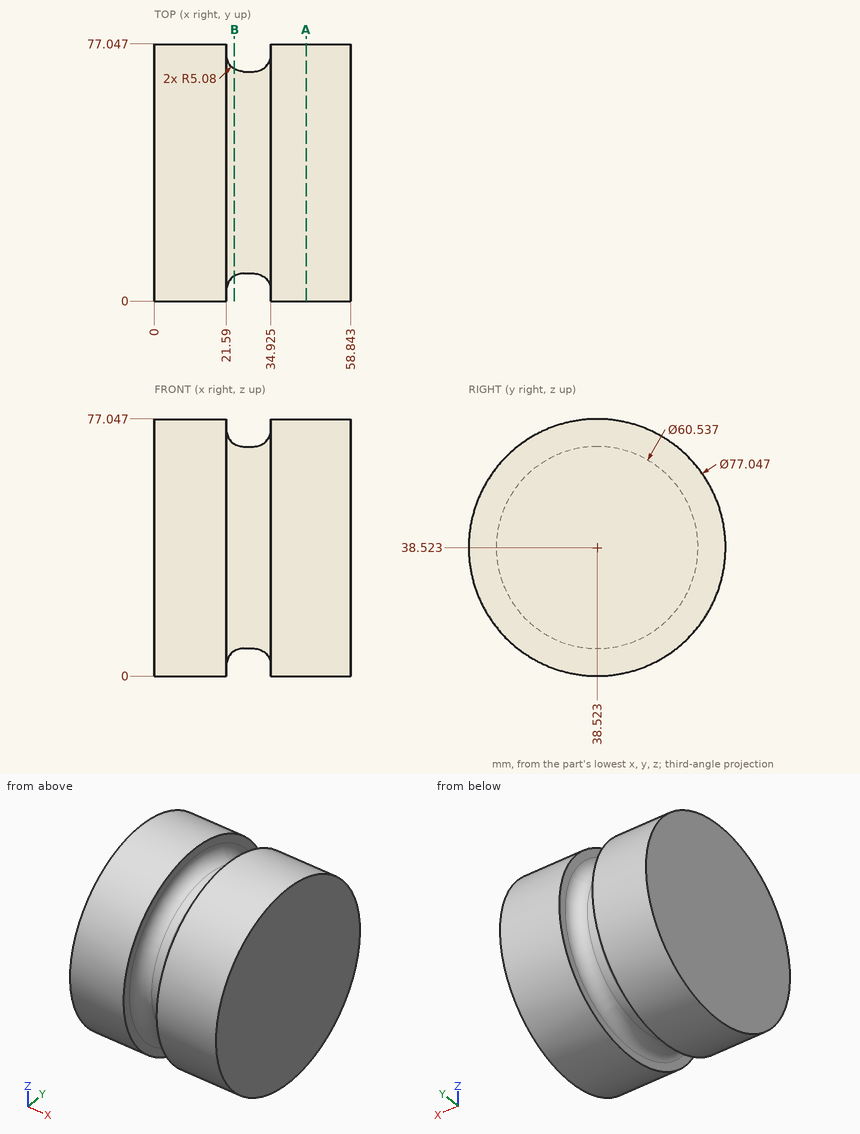
Print and shaded views of the part. All mm, measured from the part's lowest x, y and z. Give positions to 0.01 mm unless a question says otherwise; leave off trailing zeros. Write each loop counter-clockwise with the first axis right and the second up, starting at its lowest first coordinate (ties: lowest second). Pieces come first, ordered by that corner, then holes. Notation, with made-up numbers: M -15.5,59.25 L 32.5,59.25 A18 ccw 32.5,78.25 Z; hole C 23.25,14 d3. An arc over 180 degrees is marked long. Use a Markdown table: item, result.
1) Drill centre lines: line 1 (X direction, y = 70, z = 50.5); line 2 (X direction, y = 19, z = 62.5) (1 decimal); line 3 (Z direction, x = 5, y = 39). Where is each one in solid material? Low to high. Write a range as from..to.
Responses:
| item | result |
|---|---|
| line 1 | x = 0..21.87, 34.64..58.84 |
| line 2 | x = 0..24.2, 32.3..58.8 |
| line 3 | z = 0..77.04 |
2) Cut at B-B (x = 24). List the corners of the cut face in (y, z).
Responses:
| item | result |
|---|---|
| outline | C 38.52,38.52 d62.05 |
3) Cut at A-A (x = 45.5). List the corners of the cut face in (y, z), and give its area (3 significant figures).
Responses:
| item | result |
|---|---|
| outline | C 38.52,38.52 d77.05 |
| area | 4,660 mm2 |
4) Pin check, flat tips, straight feed: pin 1 (6 mm diameter, centred on x = 8, y = 63.5, fed in from -Z); pin 2 (2 mm diameter, centred on x = 9.5, z = 12.5, fed in from +Y); pin 3 (12 mm diameter, centred on x = 21.5, z = 34.5, fed in from -Y); pin 4 (6 mm diameter, centred on y = 19.5, z = 45.5, fed in from -X). Stop position of each tip, or through.
Responses:
| item | result |
|---|---|
| pin 1 | stops at z = 6.88 |
| pin 2 | stops at y = 67.81 |
| pin 3 | stops at y = 0 |
| pin 4 | stops at x = 0 |
